Verification items for the finished model (mm, model axes). Give positions to 0.01 mm unless a question says otherwise; leave off trailing zeros. Order: outer loops, then holes, each group sorted by start corner. A loop starts at its lowest first (then second) coordinate and runs counter-clockwise, first axis right, second up. Notation, with made-up numbers: (-13.75, 11) -> (34.25, 11) arc R14 cw to (34.25, 24) -> close; hole circle Ø4 at (17.5, 36). An arc over 180 degrees is marked (long way). Return JSON: item names as keys, results as strings. Group by question number.
(1) Cross-section at B-B on x = -9. Enter the section's corners in (y, z).
(2) Cross-section at A-A on z = 21. Enter the section's corners in (x, y).
(3) Thickness scan on line 1 along X through (y, z) = (6.5, 60.5); line 2 along Z through (x, y) = (1.5, 4); line 3 along X through (y, z) = (4.75, -3). Record the ranges inside material, lowest first.
(4) Depth check by flat-ended pin: pin 1 Ø5 at (x, z) = (117.5, -7.5) entering from +Y. Enter the tip coordinate at first touch or a pass-through.
(5) Cross-section at C-C on z = 40.5. Enter the section's corners in (x, y), then the cut area to 3 significant figures.
(6) Cross-section at D-D on y = 6.5. State how many separate pieces and enclosed holes the cut face has, then the cut area to 3 significant figures.
from build123d import *

# Parameters (mm, degrees)
SKETCH4_W               = 250
SKETCH4_H               = 155
BOSS_EXTRUDE2_DEPTH     = 10
SKETCH5_R               = 1.5
CUT_EXTRUDE1_DEPTH      = 10
SKETCH6_R               = 1.5
CUT_EXTRUDE2_DEPTH      = 148.415229878
CUT_EXTRUDE4_DEPTH      = 299.317469373
CUT_EXTRUDE4_DEPTH_BACK = 299.317469373
SKETCH8_R               = 12.5
SKETCH10_R              = 1.5
CUT_EXTRUDE5_DEPTH      = 148.415229878
SKETCH11_W              = 30
SKETCH11_H              = 10
CUT_EXTRUDE6_DEPTH      = 148.415229878
SKETCH12_W              = 30
SKETCH12_H              = 10
CUT_EXTRUDE7_DEPTH      = 148.415229878
SKETCH14_R              = 1.5
CUT_EXTRUDE8_DEPTH      = 148.415229878
SKETCH16_W              = 10
SKETCH16_H              = 95
CUT_EXTRUDE9_DEPTH      = 10


with BuildPart() as part:
    # Sketch4 → Boss-Extrude2 (new body)
    with BuildSketch(Plane(origin=(0, 0, 0), x_dir=(1, 0, 0), z_dir=(0, 1, 0))):
        Rectangle(SKETCH4_W, SKETCH4_H)
    extrude(amount=BOSS_EXTRUDE2_DEPTH)

    # Sketch5 → Cut-Extrude1 (cut)
    with BuildSketch(Plane.XZ):
        with Locations(Location((-110, 47.5, 0), (0, 0, 270))):
            Circle(SKETCH5_R)
    cut_extrude1 = extrude(amount=-CUT_EXTRUDE1_DEPTH, mode=Mode.SUBTRACT)

    # Mirror1: Cut-Extrude1 across plane
    add(cut_extrude1.mirror(Plane.XY), mode=Mode.SUBTRACT)

    # Sketch6 → Cut-Extrude2 (cut, symmetric)
    with BuildSketch(Plane.XZ):
        with Locations(Location((75, 14.5, 0), (0, 0, 270))):
            Circle(SKETCH6_R)
    cut_extrude2 = extrude(amount=CUT_EXTRUDE2_DEPTH, both=True, mode=Mode.SUBTRACT)

    # Mirror2: Cut-Extrude2 across plane
    add(cut_extrude2.mirror(Plane.XY), mode=Mode.SUBTRACT)

    # Sketch8 → Cut-Extrude4 (cut, two sides: drawn at the far end of the back side and taken through both)
    with BuildSketch(Plane(origin=(-47.523167836, 19.5, 165.087755447), x_dir=(1, 0, 0), z_dir=(0, 1, 0)).offset(-CUT_EXTRUDE4_DEPTH_BACK)):
        with Locations(Location((-27.476832164, 144.087755447, 0), (0, 0, 270))):
            Circle(SKETCH8_R)
        with Locations(Location((-27.476832164, 185.912244553, 0), (0, 0, 270))):
            Circle(SKETCH8_R)
    extrude(amount=CUT_EXTRUDE4_DEPTH + CUT_EXTRUDE4_DEPTH_BACK, mode=Mode.SUBTRACT)

    # Sketch10 → Cut-Extrude5 (cut, symmetric)
    with BuildSketch(Plane(origin=(0, 0, 0), x_dir=(-1, 0, 0), z_dir=(0, -1, 0))):
        with Locations(Location((75, -47.5, 0), (0, 0, 90))):
            Circle(SKETCH10_R)
    cut_extrude5 = extrude(amount=CUT_EXTRUDE5_DEPTH, both=True, mode=Mode.SUBTRACT)

    # Mirror3: Cut-Extrude5 across plane
    add(cut_extrude5.mirror(Plane.XY), mode=Mode.SUBTRACT)

    # Sketch11 → Cut-Extrude6 (cut, symmetric)
    with BuildSketch(Plane.XZ):
        with Locations((-10, 62.5)):
            Rectangle(SKETCH11_W, SKETCH11_H)
    cut_extrude6 = extrude(amount=CUT_EXTRUDE6_DEPTH, both=True, mode=Mode.SUBTRACT)

    # Sketch12 → Cut-Extrude7 (cut, symmetric)
    with BuildSketch(Plane(origin=(0, 0, 0), x_dir=(-1, 0, 0), z_dir=(0, -1, 0))):
        with Locations((-35, -62.5)):
            Rectangle(SKETCH12_W, SKETCH12_H)
    cut_extrude7 = extrude(amount=CUT_EXTRUDE7_DEPTH, both=True, mode=Mode.SUBTRACT)

    # Mirror4: Cut-Extrude6, Cut-Extrude7 across plane
    add(cut_extrude6.mirror(Plane.XY), mode=Mode.SUBTRACT)
    add(cut_extrude7.mirror(Plane.XY), mode=Mode.SUBTRACT)

    # Sketch14 → Cut-Extrude8 (cut, symmetric)
    with BuildSketch(Plane.XZ):
        with Locations(Location((117.5, 7.5, 0), (0, 0, 270))):
            Circle(SKETCH14_R)
    cut_extrude8 = extrude(amount=CUT_EXTRUDE8_DEPTH, both=True, mode=Mode.SUBTRACT)

    # Mirror5: Cut-Extrude8 across plane
    add(cut_extrude8.mirror(Plane.XY), mode=Mode.SUBTRACT)

    # Sketch16 → Cut-Extrude9 (cut)
    with BuildSketch(Plane(origin=(-47.523167836, 10, 165.087755447), x_dir=(1, 0, 0), z_dir=(0, 1, 0))):
        with Locations((107.523167836, 165.087755447)):
            Rectangle(SKETCH16_W, SKETCH16_H)
        with Locations((2.523167836, 165.087755447)):
            Rectangle(SKETCH16_W, SKETCH16_H)
    extrude(amount=-CUT_EXTRUDE9_DEPTH, mode=Mode.SUBTRACT)


solid = part.part
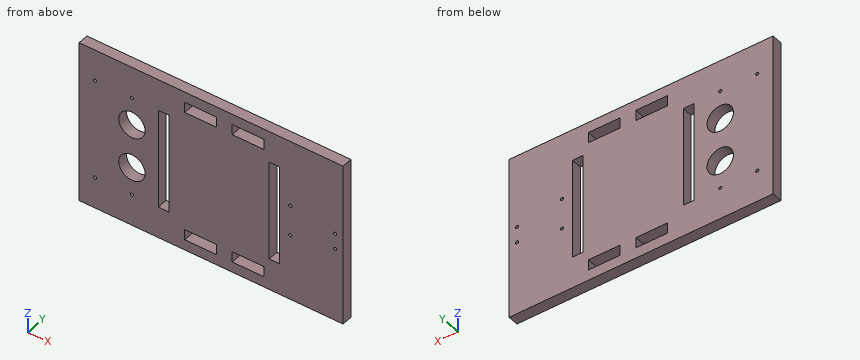
Verdict:
{
 "1": {"outline": "(0, -77.5) -> (10, -77.5) -> (10, -67.5) -> (0, -67.5) -> close; (0, -57.5) -> (10, -57.5) -> (10, 57.5) -> (0, 57.5) -> close; (0, 67.5) -> (10, 67.5) -> (10, 77.5) -> (0, 77.5) -> close"},
 "2": {"outline": "(-125, 0) -> (-87.5, 0) -> (-87.5, 10) -> (-125, 10) -> close; (-62.5, 0) -> (-50, 0) -> (-50, 10) -> (-62.5, 10) -> close; (-40, 0) -> (55, 0) -> (55, 10) -> (-40, 10) -> close; (65, 0) -> (125, 0) -> (125, 10) -> (65, 10) -> close"},
 "3": {"line 1": "-125 to -25, 5 to 20, 50 to 125", "line 2": "-77.5 to -67.5, -57.5 to 57.5, 67.5 to 77.5", "line 3": "-125 to -50, -40 to 55, 65 to 125"},
 "4": {"pin 1": "y = 10"},
 "5": {"outline": "(-125, 0) -> (-50, 0) -> (-50, 10) -> (-125, 10) -> close; (-40, 0) -> (55, 0) -> (55, 10) -> (-40, 10) -> close; (65, 0) -> (125, 0) -> (125, 10) -> (65, 10) -> close", "area": "2,300 mm²"},
 "6": {"separate pieces": "1", "enclosed holes": "16", "area": "34,600 mm²"}
}
